Here's how the part is built. I have some questions about the finished solid (model axes, mm). Round coordinates to 2 decimals unless told otherwise and drop trailing zeros. Loops run counter-clockwise (first coordinate to the right, second up) from the corner with the lowest first, then second, coordinate; pieces in that order, holes last. Notation, with made-up numbers: M -29.5,25.25 L -9.5,25.25 A11 ccw -9.5,38.25 Z; hole C 50,55 d9. An arc over 180 degrees is marked long. Put each result on its own line as item: value. Start each with the question number.
```python
from build123d import *

# Parameters (mm, degrees)
BOSS_EXTRUDE1_DEPTH = 9.525
CUT_EXTRUDE1_DEPTH  = 9.525


with BuildPart() as part:
    # Sketch1 → Boss-Extrude1 (new body)
    with BuildSketch(Plane(origin=(0, 0, 0), x_dir=(1, 0, 0), z_dir=(0, 1, 0))):
        Polygon((0, 0), (0, 49.751846715), (-7.9375, 63.5), (-9.525, 63.5), (-9.525, 0), align=None)
    extrude(amount=BOSS_EXTRUDE1_DEPTH)

    # Sketch2 → Cut-Extrude1 (cut)
    with BuildSketch(Plane(origin=(0, 0, 0), x_dir=(0, 0, -1), z_dir=(1, 0, 0))):
        Polygon((63.5, 9.525), (61.820485509, 0), (63.5, 0), align=None)
    extrude(amount=-CUT_EXTRUDE1_DEPTH, mode=Mode.SUBTRACT)


solid = part.part
```
1) Suppose I cut it at C-C (z = -59). Write out the boundary of the cut face in (x, y) (3 decimals), plus the area to 3 significant figures.
2) Suppose I cut it at A-A (y = 3.5). Write out the boundary of the cut face in (x, z) (3 decimals), plus the area to 3 significant figures.
3) If I drill on probe 1 along Z at (x, y) = (-2.25, 1.75); probe 2 along Z at (x, y) = (-8, 1.25); probe 3 along X at (y, z) = (1.5, -52) (3 decimals), over which ranges is the centre line in solid material (lowest first)? Write a range as from..to.
4) Suppose I cut it at B-B (x = -5.5). Write out the boundary of the cut face in (y, z) (3 decimals).
5) Suppose I cut it at D-D (y = 1). Write out the boundary of the cut face in (x, z) (3 decimals), plus the area to 3 significant figures.
Results are:
1. outline: M -9.525,0 L -5.339,0 L -5.339,9.525 L -9.525,9.525 Z
1. area: 39.9 mm²
2. outline: M -9.525,-62.438 L -7.324,-62.438 L 0,-49.752 L 0,0 L -9.525,0 Z
2. area: 548 mm²
3. probe 1: -53.65..0
3. probe 2: -62.04..0
3. probe 3: -9.525..-1.298
4. outline: M 0,-59.278 L 9.525,-59.278 L 9.525,0 L 0,0 Z
5. outline: M -9.525,-61.997 L -7.07,-61.997 L 0,-49.752 L 0,0 L -9.525,0 Z
5. area: 547 mm²
